Could you check a few things on this drawing? It's one solid part, dimensions in mm from its lowest x, y, z. Round coordinates to 2 decimals unless told otherwise and drop trailing zeros. Loops run counter-clockwise (first coordinate to the right, second up) from the corner with the lowest first, then second, coordinate; pieces in that order, holes last. Notation, with made-up numbers: M 81.25,-13.5 L 89.25,-13.5 A25 ccw 89.25,22.5 Z; hole C 81,29 d5. An arc over 180 degrees is marked long. Use a Markdown table: item, result. Add a question column.
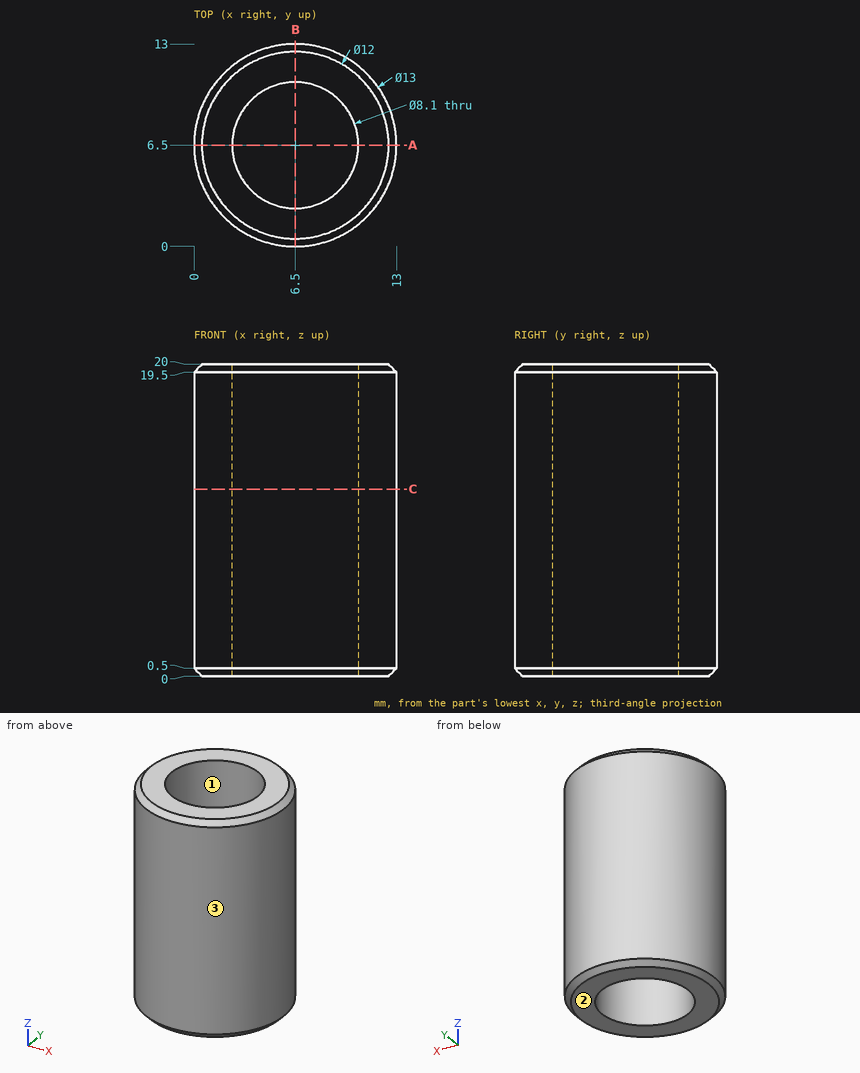
(1) I'm going to push flat-ended pins straight in: pin 1 (6 mm diameter, centred on x = 1.5, z = 17, fed in from +Y); pin 2 (5 mm diameter, centred on y = 9.5, z = 10, fed in from +X); pin 3 (2 mm diameter, centred on y = 8.5, z = 10, fed in from +X). Where does each tip first touch, or does it pass through?
(2) Suppose I cut it at C-C on z = 12. List the corners of the cut face in (x, y) for me.
(3) Thinking about a two-plate mould opening in X: for the marked faces 1, 2 and 3, which applies, released by +X, released by -X, zero draft, split by the parting line, or undercut?
(4) Suppose I cut it at A-A on y = 6.5. List the corners of the cut face in (x, z) for me, and give its area (3 significant figures).
(5) If I drill on probe 1 along Y at (x, z) = (6.5, 4); probe 2 along X at (y, z) = (4, 11.25), over which ranges is the centre line in solid material (lowest first)? Write a range as [from, to].
Results below:
| question | item | result |
|---|---|---|
| 1 | pin 1 | stops at y = 12.68 |
| 1 | pin 2 | stops at x = 12.98 |
| 1 | pin 3 | stops at x = 12.92 |
| 2 | outline | C 6.5,6.5 d13; hole C 6.5,6.5 d8.1 |
| 3 | face 1 | undercut |
| 3 | face 2 | zero draft |
| 3 | face 3 | split by the parting line |
| 4 | outline | M 0,0.5 L 0.5,0 L 2.45,0 L 2.45,20 L 0.5,20 L 0,19.5 Z; M 10.55,0 L 12.5,0 L 13,0.5 L 13,19.5 L 12.5,20 L 10.55,20 Z |
| 4 | area | 97.5 mm² |
| 5 | probe 1 | y = [0, 2.45], [10.55, 13] |
| 5 | probe 2 | x = [0.5, 3.31], [9.69, 12.5] |
